from build123d import *

# Parameters (mm, degrees)
SKETCH1_W             = 7.7
SKETCH1_H             = 6
BOSS_EXTRUDE1_DEPTH   = 8
SKETCH2_W             = 2.5
SKETCH2_H             = 6
CUT_EXTRUDE1_DEPTH    = 6
F_3_0MM_DOWEL_HOLE1_D = 3
SKETCH7_W             = 15
SKETCH7_H             = 6
BOSS_EXTRUDE2_DEPTH   = 2
M3_CLEARANCE_HOLE1_D  = 3.2
FILLET1_R             = 2
FILLET2_R             = 1


with BuildPart() as part:
    # Sketch1 → Boss-Extrude1 (new body)
    with BuildSketch(Plane(origin=(0, 0, 0), x_dir=(1, 0, 0), z_dir=(0, 1, 0))):
        with Locations((3.85, 3)):
            Rectangle(SKETCH1_W, SKETCH1_H)
    extrude(amount=BOSS_EXTRUDE1_DEPTH)

    # Sketch2 → Cut-Extrude1 (cut)
    with BuildSketch(Plane(origin=(0, 8, 0), x_dir=(1, 0, 0), z_dir=(0, 1, 0))):
        with Locations((3.85, 3)):
            Rectangle(SKETCH2_W, SKETCH2_H)
    extrude(amount=-CUT_EXTRUDE1_DEPTH, mode=Mode.SUBTRACT)

    # Ø3.0mm Dowel Hole1 (through all)
    with Locations(Plane.ZY):
        with Locations((-3, 5)):
            Hole(F_3_0MM_DOWEL_HOLE1_D / 2)

    # Sketch7 → Boss-Extrude2 (add)
    with BuildSketch(Plane.XZ):
        with Locations((3.85, -9)):
            Rectangle(SKETCH7_W, SKETCH7_H)
    extrude(amount=-BOSS_EXTRUDE2_DEPTH)

    # M3 Clearance Hole1 (through all)
    with Locations(Plane(origin=(0, 2, 0), x_dir=(1, 0, 0), z_dir=(0, 1, 0))):
        with Locations((-0.65, 9), (8.35, 9)):
            Hole(M3_CLEARANCE_HOLE1_D / 2)

    # Fillet1
    fillet1_edges = [part.edges().sort_by_distance(p)[0] for p in [
        (6.4, 8, 0),
        (1.3, 8, -6),
        (6.4, 8, -6),
        (-3.65, 1, -6),
        (-3.65, 1, -12),
        (11.35, 1, -6),
        (11.35, 1, -12),
        (1.3, 8, 0),
    ]]
    fillet(fillet1_edges, radius=FILLET1_R)

    # Fillet2
    # the kernel refuses this fillet: 1 mm, written as the material it takes off along each edge
    with BuildSketch(Plane(origin=(7.7, -2.5, 0), x_dir=(-1, 0, 0), z_dir=(0, 1, 0))) as fillet2_piece_1:
        with BuildLine():
            CenterArc((FILLET2_R, -FILLET2_R), FILLET2_R, 90, 90)
            Line((0, -FILLET2_R), (0, 0))
            Line((0, 0), (FILLET2_R, 0))
        make_face()
    extrude(amount=11, mode=Mode.SUBTRACT)


solid = part.part
Read the model definition and answer for the solid it produces. Units are mm, in the model's axes. A direction names the side the tool comes from. Round coordinates to 2 decimals unless told otherwise and drop trailing zeros. Write each loop counter-clockwise with the first axis right and the second up, starting at its lowest first coordinate (ties: lowest second). Pieces come first, ordered by that corner, then holes. Notation, with made-up numbers: (35, 35.25) - (81, 35.25) arc R20 ccw to (81, 39.25) - close; hole circle Ø3 at (29, 21). An arc over 180 degrees is marked (long way). One line per question, with ' | ' between items. Start each with the question number.
1. Section C-C (x = 8.35) is taken. Determine the outline of the cut face in (y, z).
2. Find the intervals of material crossed by probe 1 along X at (y, z) = (1.4, -9); probe 2 along Y at (x, z) = (1.75, -3); probe 3 along X at (y, z) = (7.25, -4.5), in increasing order. Write a range as [from, to].
3. Each of these flat-tipped pins is pushed along its axis until it touches: pin 1 (1.5 mm diameter, centred on y = 2, z = -3, fed in from +X); pin 2 (5 mm diameter, centred on x = 8.35, z = -9, fed in from +Y); pin 3 (2 mm diameter, centred on x = 0.5, y = 4.5, fed in from -Z); pin 4 (1.8 mm diameter, centred on y = 5, z = -3, fed in from -X). Where does it stop, or does it pass through?
4. Section D-D (y = 0.5) is taken. Determine the outline of the cut face in (x, z), and give its area (3 significant figures).
5. Section A-A (z = -3) is taken. Determine the outline of the cut face in (x, y).
6. For faces 1 (the face through (2.6, 3.7, -4.3)), 2 (the face through (7.7, 3, -3)), 3 (the face through (8.7, 0.99, -7.44)), 4 (the face through (0, 3, -3)), determine the directions among +Z, -Z, +X, -X, +Y, -Y from which every point of the face is accessible in a straight line to the end or side of a thin tool.
7. Section B-B (y = 5) is taken. Determine the outline of the cut face in (x, z).
8. For a pull along Y with two mould halves and no side action, classify faces 5 (the face through (6.42, 7.4, -0.57)), 6 (the face through (-3.65, 1, -9)), 7 (the face through (6.418, 4.425, -4.386)) as +Y half, -Y half, draft (parallel to the pull), parting line (faces both ways), or undercut.
Filled in:
1) outline: (0, -12) - (2, -12) - (2, -10.6) - (0, -10.6) - close; (0, -7.4) - (2, -7.4) - (2, -6) - (0, -6) - close
2) probe 1: [-3.65, -2.25], [0.95, 6.75], [9.95, 11.35] | probe 2: [0, 3.5], [6.5, 8] | probe 3: [0, 2.6], [5.1, 7.7]
3) pin 1: x = 7.7 | pin 2: y = 2 | pin 3: z = -6 | pin 4: through
4) outline: (-3.65, -10) arc R2 ccw to (-1.65, -12) - (9.35, -12) arc R2 ccw to (11.35, -10) - (11.35, -8) arc R2 ccw to (9.35, -6) - (7.7, -6) - (7.7, -1) arc R1 ccw to (6.7, 0) - (0, 0) - (0, -6) - (-1.65, -6) arc R2 ccw to (-3.65, -8) - close; hole circle Ø3.2 at (-0.65, -9); hole circle Ø3.2 at (8.35, -9) | area: 116 mm²
5) outline: (0, 0) - (7.7, 0) - (7.7, 3.5) - (5.1, 3.5) - (5.1, 2) - (2.6, 2) - (2.6, 3.5) - (0, 3.5) - close; (0, 6.5) - (2.6, 6.5) - (2.6, 8) - (0, 8) - close; (5.1, 6.5) - (7.7, 6.5) - (7.7, 8) - (5.1, 8) - close
6) face 1: +Z, -Z, +Y | face 2: +Z, +X, +Y, -Y | face 3: +Y, -Y | face 4: +Z, -X, +Y, -Y
7) outline: (0, -6) - (2.6, -6) - (2.6, -4.5) - (0, -4.5) - close; (0, -1.5) - (2.6, -1.5) - (2.6, 0) - (0, 0) - close; (5.1, -6) - (7.7, -6) - (7.7, -4.5) - (5.1, -4.5) - close; (5.1, -1.5) - (7.7, -1.5) - (7.7, -1) arc R1 ccw to (6.7, 0) - (5.1, 0) - close
8) face 5: +Y half | face 6: draft | face 7: undercut
